```python
from build123d import *

# Parameters (mm, degrees)
SKETCH_W             = 43
SKETCH_H             = 21
SKETCH_R             = 1.5
PAD_DEPTH            = 1.5
SKETCH001_R          = 4
PAD001_DEPTH         = 10
FILLET_R             = 1
SKETCH002_W          = 12
SKETCH002_H          = 12
PAD002_DEPTH         = 7
FILLET001_R          = 2
SKETCH003_W          = 9
SKETCH003_H          = 4
PAD003_DEPTH         = 10
SKETCH004_R          = 1
PAD004_DEPTH         = 1
SKETCH005_W          = 9
SKETCH005_H          = 7
PAD005_DEPTH         = 3
SKETCH006_W          = 4
SKETCH006_H          = 2
PAD006_DEPTH         = 2
BODY_PLACEMENT_ANGLE = 180


with BuildPart() as part:
    # Sketch → Pad (new body)
    with BuildSketch(Plane.XZ):
        with Locations((21.5, 10.5)):
            Rectangle(SKETCH_W, SKETCH_H)
        with Locations((6.5, 18.5)):
            Circle(SKETCH_R, mode=Mode.SUBTRACT)
        with Locations((36.5, 2.5)):
            Circle(SKETCH_R, mode=Mode.SUBTRACT)
    extrude(amount=PAD_DEPTH)

    # Sketch001 (on Face8 of Pad) → Pad001 (join)
    with BuildSketch(Plane.XZ.offset(1.5)):
        with Locations((5, 10.5)):
            Circle(SKETCH001_R)
        with Locations((38, 10.5)):
            Circle(SKETCH001_R)
    extrude(amount=PAD001_DEPTH)

    # Fillet
    fillet_edges = [part.edges().sort_by_distance(p)[0] for p in [
        (1, -11.5, 10.5),
        (34, -11.5, 10.5),
    ]]
    fillet(fillet_edges, radius=FILLET_R)

    # Sketch002 (on Face3 of Fillet) → Pad002 (join)
    with BuildSketch(Plane.XZ.offset(1.5)):
        with Locations((16, 14)):
            Rectangle(SKETCH002_W, SKETCH002_H)
    extrude(amount=PAD002_DEPTH)

    # Fillet001
    fillet001_edges = [part.edges().sort_by_distance(p)[0] for p in [
        (22, -5, 20),
        (22, -5, 8),
        (10, -5, 20),
        (10, -5, 8),
    ]]
    fillet(fillet001_edges, radius=FILLET001_R)

    # Sketch003 (on Face1 of Fillet001) → Pad003 (join)
    with BuildSketch(Plane.XZ.offset(1.5)):
        with Locations((14.5, 3.5)):
            Rectangle(SKETCH003_W, SKETCH003_H)
    extrude(amount=PAD003_DEPTH)

    # Sketch004 (on Face25 of Pad003) → Pad004 (join)
    with BuildSketch(Plane.XZ.offset(11.5)):
        with Locations((17.5, 3)):
            Circle(SKETCH004_R)
    extrude(amount=PAD004_DEPTH)

    # Sketch005 (on Face1 of Pad004) → Pad005 (join)
    with BuildSketch(Plane.XZ.offset(1.5)):
        with Locations((27.5, 5.5)):
            Rectangle(SKETCH005_W, SKETCH005_H)
    extrude(amount=PAD005_DEPTH)

    # Sketch006 (on Face1 of Pad005) → Pad006 (join)
    with BuildSketch(Plane.XZ.offset(1.5)):
        with Locations((29, 19)):
            Rectangle(SKETCH006_W, SKETCH006_H)
    extrude(amount=PAD006_DEPTH)


with BuildPart() as part_1:
    # Body placement: moved
    add(part.part.rotate(Axis((0, 0, 0), (1, 0, 0)), BODY_PLACEMENT_ANGLE))


solid = part_1.part
```
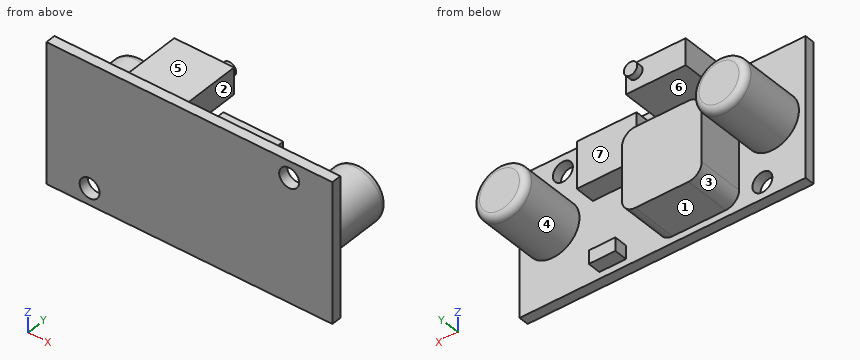
For this review, take the finished solid that the model builds, in its own axes (mm). Face numbers are marked on the shaded views. A direction names the side the tool comes from. Coordinates: 2 decimals unless noted, no trailing zeros. Loops run counter-clockwise (first coordinate to the right, second up) from the corner with the lowest first, then second, coordinate; pieces in that order, holes last.
1. Add section C-C, the plane z = -4.75. Give the boundary of the cut face in (x, y), then the cut area to 4 significant figures.
2. Add section B-B, the plane x = 17.5. Give the boundary of the cut face in (y, z), then the cut area to 4 significant figures.
3. Mouldability with a two-part tool opening along X and no side actions: class the marked faces 1, 2 and 3 as +X half, -X half, draft (parallel to the pull), parting line (faces both ways), or undercut.
4. For line 1 (X direction, y = 6, z = -10.5); line 2 (Z direction, x = 36.5, y = 0.45); line 3 (X direction, y = 0.45, z = -18.5), list the stretches that pass through material, from the lowest coordinate up.
5. Add section D-D, the plane z = -2.5. Give the boundary of the cut face in (x, y).
6. Insertion check: P1, Ø3, axis at x = 20, z = -14, coming from the +Y side; P2, Ø0.9, axis at y = 2.5, z = -5, coming from the -X side; P3, Ø2, axis at x = 29, z = -19, coming from the +Y side; P4, Ø3.5, axis at y = 2.5, z = -6, coming from the +X side. Each pin has a flat end and moves straight along its axis. Give the tip position at first contact, or say it passes through.
7. For the marked faces 4, 5, 6 and 7, list the 3-axis set-ups (+Z, -Z, +X, -X, +Y, -Y) from which the entire face can be reached by the end or side of a thin tool; tool diameter is ignored.
8. Add section A-A, the plane z = -18.5. Give the boundary of the cut face in (x, y).
Result:
1. outline: (0, 0) - (43, 0) - (43, 1.5) - (32, 1.5) - (32, 4.5) - (23, 4.5) - (23, 1.5) - (19, 1.5) - (19, 11.5) - (10, 11.5) - (10, 1.5) - (0, 1.5) - close
1. area: 181.5 mm2
2. outline: (0, -21) - (1.5, -21) - (1.5, -20) - (8.5, -20) - (8.5, -8) - (1.5, -8) - (1.5, -5.5) - (11.5, -5.5) - (11.5, -4) - (12.5, -4) - (12.5, -2) - (11.5, -2) - (11.5, -1.5) - (1.5, -1.5) - (1.5, 0) - (0, 0) - close
2. area: 157.5 mm2
3. face 1: draft
3. face 2: undercut
3. face 3: -X half
4. line 1: x = 1 to 9, 10 to 22, 34 to 42
4. line 2: z = -21 to -4, -1 to 0
4. line 3: x = 0 to 5, 8 to 43
5. outline: (0, 0) - (35, 0) - (35, 1.5) - (32, 1.5) - (32, 4.5) - (23, 4.5) - (23, 1.5) - (19, 1.5) - (19, 11.5) - (18.37, 11.5) - (18.37, 12.5) - (16.63, 12.5) - (16.63, 11.5) - (10, 11.5) - (10, 1.5) - (0, 1.5) - close; (38, 0) - (43, 0) - (43, 1.5) - (38, 1.5) - close
6. P1: stops at y = 8.5
6. P2: stops at x = 10
6. P3: stops at y = 3.5
6. P4: stops at x = 43
7. face 4: +Y
7. face 5: +Z, +X, -X, +Y
7. face 6: -X, +Y
7. face 7: +Z, -Z, +Y
8. outline: (0, 0) - (5, 0) - (5, 1.5) - (0, 1.5) - close; (8, 0) - (43, 0) - (43, 1.5) - (31, 1.5) - (31, 3.5) - (27, 3.5) - (27, 1.5) - (21.94, 1.5) - (21.94, 8.5) - (10.06, 8.5) - (10.06, 1.5) - (8, 1.5) - close
